from build123d import *

# Parameters (mm, degrees)
F0_R        = 0.635
F0_R_2      = 0.762
F1_DEPTH    = 2.54
F2_T1_DEPTH = 19.2320747894
F2_T3_DEPTH = 54.1570747894


# Not quite as in the source:
# - a fillet or chamfer that OpenCascade refuses, or shapes differently, is made with other operations: its cross-section is extruded or revolved along the edge and cut away or added


with BuildPart() as f1:
    # F0 (on Front) → F1 (new body)
    with BuildSketch(Plane.XZ):
        Polygon((44.45, 12.7), (0, 12.7), (-3.175, 12.7), (-3.175, 0), (0, 0), (44.45, 0), align=None)
        with Locations((3.1763850711, 1.8884516321)):
            Circle(F0_R, mode=Mode.SUBTRACT)
        with BuildLine():
            ThreePointArc((12.7013850711, 1.8884516321), (12.0663850711, 1.2534516321), (11.4313850711, 1.8884516321))
            ThreePointArc((11.4313850711, 1.8884516321), (12.0663850711, 2.5234516321), (12.7013850711, 1.8884516321))
        make_face(mode=Mode.SUBTRACT)
        with Locations((0, 6.35)):
            Circle(F0_R_2, mode=Mode.SUBTRACT)
        with BuildLine():
            ThreePointArc((3.9569724428, 5.2575343288), (2.8729596367, 4.8085215228), (3.3219724428, 5.8925343288))
            ThreePointArc((3.3219724428, 5.8925343288), (3.7709852488, 5.7065471349), (3.9569724428, 5.2575343288))
        make_face(mode=Mode.SUBTRACT)
        with BuildLine():
            ThreePointArc((25.4013850711, 1.8884516321), (24.7663850711, 1.2534516321), (24.1313850711, 1.8884516321))
            ThreePointArc((24.1313850711, 1.8884516321), (24.7663850711, 2.5234516321), (25.4013850711, 1.8884516321))
        make_face(mode=Mode.SUBTRACT)
        with BuildLine():
            ThreePointArc((30.3330272979, 3.1118398262), (29.2490144918, 2.6628270202), (29.6980272979, 3.7468398262))
            ThreePointArc((29.6980272979, 3.7468398262), (30.1470401039, 3.5608526323), (30.3330272979, 3.1118398262))
        make_face(mode=Mode.SUBTRACT)
        with BuildLine():
            ThreePointArc((36.7843080854, 2.629004186), (35.7002952794, 2.17999138), (36.1493080854, 3.264004186))
            ThreePointArc((36.1493080854, 3.264004186), (36.5983208915, 3.0780169921), (36.7843080854, 2.629004186))
        make_face(mode=Mode.SUBTRACT)
        with BuildLine():
            ThreePointArc((25.2530272979, 4.8898398262), (24.1690144918, 4.4408270202), (24.6180272979, 5.5248398262))
            ThreePointArc((24.6180272979, 5.5248398262), (25.0670401039, 5.3388526323), (25.2530272979, 4.8898398262))
        make_face(mode=Mode.SUBTRACT)
        with BuildLine():
            ThreePointArc((27.7930272979, 4.8898398262), (27.1580272979, 4.2548398262), (26.5230272979, 4.8898398262))
            ThreePointArc((26.5230272979, 4.8898398262), (26.7090144918, 5.3388526323), (27.1580272979, 5.5248398262))
            ThreePointArc((27.1580272979, 5.5248398262), (27.6070401039, 5.3388526323), (27.7930272979, 4.8898398262))
        make_face(mode=Mode.SUBTRACT)
        with BuildLine():
            ThreePointArc((36.7843080854, 5.118204186), (36.5983208915, 4.66919138), (36.1493080854, 4.483204186))
            ThreePointArc((36.1493080854, 4.483204186), (35.7002952794, 5.5672169921), (36.7843080854, 5.118204186))
        make_face(mode=Mode.SUBTRACT)
        with Locations((39.9367623031, 6.35)):
            Circle(F0_R_2, mode=Mode.SUBTRACT)
        with BuildLine():
            ThreePointArc((3.3219724428, 7.1625343288), (2.6869724428, 7.7975343288), (3.3219724428, 8.4325343288))
            ThreePointArc((3.3219724428, 8.4325343288), (3.7709852488, 8.2465471349), (3.9569724428, 7.7975343288))
            ThreePointArc((3.9569724428, 7.7975343288), (3.7709852488, 7.3485215228), (3.3219724428, 7.1625343288))
        make_face(mode=Mode.SUBTRACT)
        with BuildLine():
            ThreePointArc((21.1654724428, 7.7975343288), (19.3239724428, 5.9560343288), (17.4824724428, 7.7975343288))
            ThreePointArc((17.4824724428, 7.7975343288), (19.3239724428, 9.6390343288), (21.1654724428, 7.7975343288))
        make_face(mode=Mode.SUBTRACT)
        with BuildLine():
            ThreePointArc((3.3219724428, 9.7025343288), (2.8729596367, 10.7865471349), (3.9569724428, 10.3375343288))
            ThreePointArc((3.9569724428, 10.3375343288), (3.7709852488, 9.8885215228), (3.3219724428, 9.7025343288))
        make_face(mode=Mode.SUBTRACT)
        with BuildLine():
            ThreePointArc((25.2530272979, 9.9698398262), (25.0670401039, 9.5208270202), (24.6180272979, 9.3348398262))
            ThreePointArc((24.6180272979, 9.3348398262), (24.1690144918, 10.4188526323), (25.2530272979, 9.9698398262))
        make_face(mode=Mode.SUBTRACT)
        with BuildLine():
            ThreePointArc((27.7930272979, 9.9698398262), (27.6070401039, 9.5208270202), (27.1580272979, 9.3348398262))
            ThreePointArc((27.1580272979, 9.3348398262), (26.7090144918, 10.4188526323), (27.7930272979, 9.9698398262))
        make_face(mode=Mode.SUBTRACT)
        with BuildLine():
            ThreePointArc((29.6980272979, 9.3348398262), (29.2490144918, 9.5208270202), (29.0630272979, 9.9698398262))
            ThreePointArc((29.0630272979, 9.9698398262), (29.6980272979, 10.6048398262), (30.3330272979, 9.9698398262))
            ThreePointArc((30.3330272979, 9.9698398262), (30.1470401039, 9.5208270202), (29.6980272979, 9.3348398262))
        make_face(mode=Mode.SUBTRACT)
    extrude(amount=F1_DEPTH)

    # F2: chamfer of 1.27 on 4 edges, made by hand

    # F2_s2 → F2_t1 (cut)
    with BuildSketch(Plane.XY.offset(-3.2660373947)):
        Polygon((43.18, 0), (44.45, -1.27), (44.45, 0), align=None)
        Polygon((-1.905, 0), (-3.175, -1.27), (-3.175, 0), align=None)
    extrude(amount=F2_T1_DEPTH, mode=Mode.SUBTRACT)

    # F2_s4 → F2_t3 (cut)
    with BuildSketch(Plane.YZ.offset(-6.4410373947)):
        Polygon((-1.27, 12.7), (0, 11.43), (0, 12.7), align=None)
        Polygon((0, 1.27), (-1.27, 0), (0, 0), align=None)
    extrude(amount=F2_T3_DEPTH, mode=Mode.SUBTRACT)


solid = f1.part
Here's how the part is built. I have some questions about the finished solid (model axes, mm). Coordinates: 2 decimals unless noted, no trailing zeros. Order: outer loops, then holes, each group sorted by start corner. A loop starts at its lowest first (then second) coordinate and runs counter-clockwise, first axis right, second up. Notation, with made-up numbers: (-14, -31.5) -> (9, -31.5) arc R21 ccw to (9, -13.5) -> close; hole circle Ø9 at (64, 19). An arc over 180 degrees is marked (long way). Answer in a Markdown table with one row per item.
(1) I want a section at B-B on y = -1.85. Count the separate pieces of the cut face and the enclosed holes in it, then the cut area to 3 significant figures.
Answer key:
| item | result |
|---|---|
| separate pieces | 1 |
| enclosed holes | 17 |
| area | 573 mm^2 |
(2) Thinking about a two-plate mould opening in X: for faces 1 (the face through (12.7, -1.3, 1.9)), 2 (the face through (20, 0, 5)), 3 (the face through (44.45, -2, 6)), which applies, +X half, -X half, draft (parallel to the pull), parting line (faces both ways), or undercut?
Answer key:
| item | result |
|---|---|
| face 1 | undercut |
| face 2 | draft |
| face 3 | +X half |
(3) Please list where these lines run through material, in increasing order: probe 1 along X at (y, z) = (-1.15, 10.5) (3 decimals); probe 2 along Z at (x, y) = (27, -0.1); probe 3 along X at (y, z) = (-0.9, 6.5) (3 decimals).
Answer key:
| item | result |
|---|---|
| probe 1 | -3.055 to 2.708, 3.936 to 24.269, 24.968 to 26.809, 27.508 to 29.349, 30.048 to 44.33 |
| probe 2 | 1.17 to 4.27, 5.5 to 9.35, 10.58 to 11.53 |
| probe 3 | -2.805 to -0.747, 0.747 to 18.017, 20.631 to 39.19, 40.684 to 44.08 |
(4) Will this pin go through, and if not, where does the flat tip stop? pin 1 Ø1 at (x, z) = (3.32, 10.34) entering from -Y.
Answer key:
| item | result |
|---|---|
| pin 1 | through |
(5) I want a section at A-A on x = 0. List the corners of the cut face in (y, z) for me, then the cut area to 3 significant figures.
Answer key:
| item | result |
|---|---|
| outline | (-2.54, 0) -> (-1.27, 0) -> (0, 1.27) -> (0, 5.59) -> (-2.54, 5.59) -> close; (-2.54, 7.11) -> (0, 7.11) -> (0, 11.43) -> (-1.27, 12.7) -> (-2.54, 12.7) -> close |
| area | 26.8 mm^2 |
